For this review, use the dimensioned drawing (mm, ordinates from the lowest corner) and the shaded views. Round coordinates to 2 decimals unless told otherwise and drop trailing zeros. Loops run counter-clockwise (first coordinate to the right, second up) from the corner with the lowest first, then second, coordinate; pieces in that order, holes last. Notation, with made-up numbers: (-31, -16.5) -> (15, -16.5) arc R15 ccw to (15, -8.5) -> close; hole circle Ø2 at (-19, 23.5). An arc over 180 degrees is marked (long way). Answer as CSV lines item,"result". Start each with the question number.
(1) To check wall thickness, follow line 1 (X direction, y = 13, z = 20.5) (1 decimal); line 2 (Y direction, x = 41.5, z = 25.5); line 3 (X direction, y = 25, z = 19). State the ranges of each line that lie inside material, in increasing order. Write a range as from..to.
(2) Draft analysis for pull direction Y (two halves, no side actions). For the marked faces 1, 2 and 3, state which applies: +Y half, -Y half, draft (parallel to the pull), parting line (faces both ways), or undercut.
(3) Take a section at D-D, the plane z = 37.5. Write out the cut boundary in (x, y) (1 decimal).
(4) Take a section at A-A, the plane x = 18.5. Write out the cut boundary in (y, z) (1 decimal).
(5) For P1, Ø8, axis at x = 12.53, y = 12.53, coming from the +Z side; P2, Ø4, axis at x = 12.53, y = 40.82, coming from the -Z side; P3, Ø6, axis at x = 40.82, y = 12.53, coming from the -Z side; P4, Ø10, axis at x = 19.5, z = 39.5, coming from the +Y side (1 decimal), all flat-tipped, find the tip position at first contact; note any pin that passes through.
(6) Take a section at C-C, the plane x = 12.5. Write out the cut boundary in (y, z) (1 decimal), and give its area (3 significant figures).
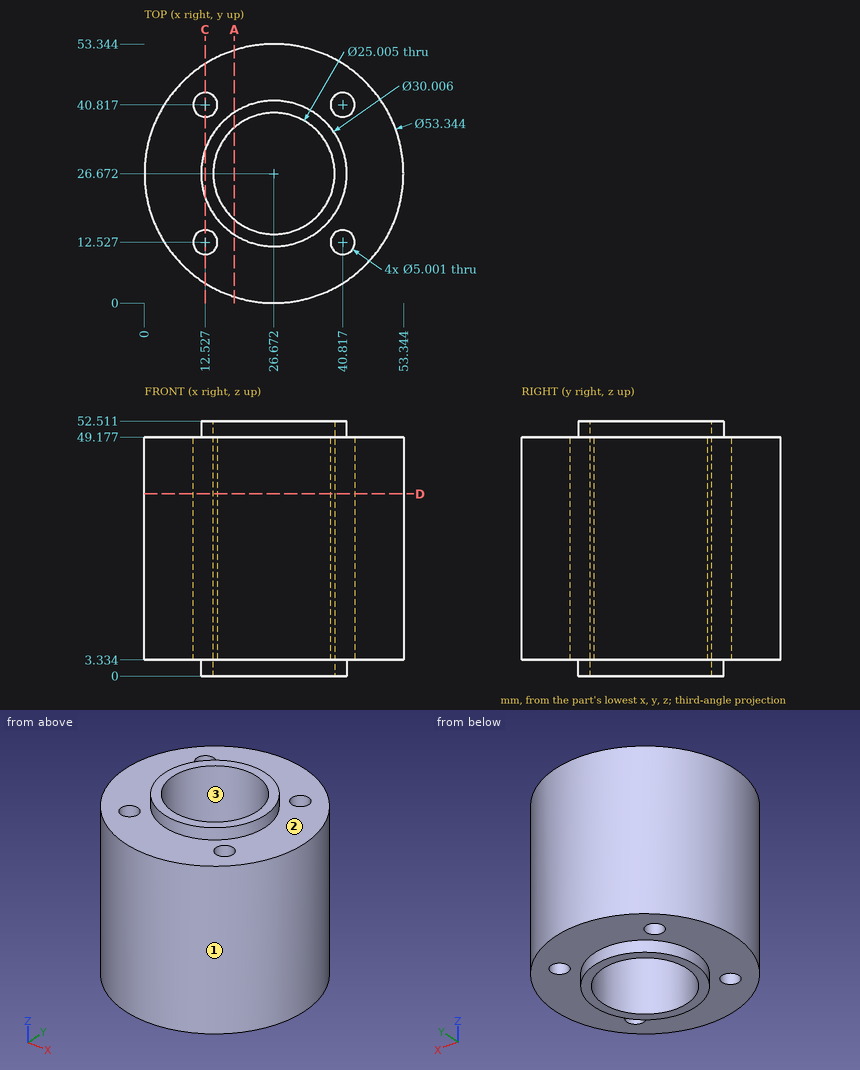
The answers:
1,line 1,"3.8..10.1, 15..38.4, 43.3..49.6"
1,line 2,"4.5..10.12, 14.93..38.41, 43.22..48.84"
1,line 3,"0.05..14.28, 39.06..53.29"
2,face 1,"parting line"
2,face 2,"draft"
2,face 3,"undercut"
3,outline,"circle Ø53.3 at (26.7, 26.7); hole circle Ø5 at (12.5, 12.5); hole circle Ø5 at (12.5, 40.8); hole circle Ø25 at (26.7, 26.7); hole circle Ø5 at (40.8, 12.5); hole circle Ø5 at (40.8, 40.8)"
4,outline,"(1.3, 3.3) -> (14.1, 3.3) -> (14.1, 0) -> (17.2, 0) -> (17.2, 52.5) -> (14.1, 52.5) -> (14.1, 49.2) -> (1.3, 49.2) -> close; (36.1, 0) -> (39.3, 0) -> (39.3, 3.3) -> (52.1, 3.3) -> (52.1, 49.2) -> (39.3, 49.2) -> (39.3, 52.5) -> (36.1, 52.5) -> close"
5,P1,"z = 49.18"
5,P2,"through"
5,P3,"z = 3.33"
5,P4,"y = 53.3"
6,outline,"(4.1, 3.3) -> (10, 3.3) -> (10, 49.2) -> (4.1, 49.2) -> close; (15, 3.3) -> (21.7, 3.3) -> (21.7, 0) -> (31.6, 0) -> (31.6, 3.3) -> (38.3, 3.3) -> (38.3, 49.2) -> (31.6, 49.2) -> (31.6, 52.5) -> (21.7, 52.5) -> (21.7, 49.2) -> (15, 49.2) -> close; (43.3, 3.3) -> (49.3, 3.3) -> (49.3, 49.2) -> (43.3, 49.2) -> close"
6,area,"1,680 mm²"
